Geometry check sheet. Reference: the model listing, model coordinates, mm. A direction names the side the tool comes from. Round coordinates to 2 decimals unless told otherwise and drop trailing zeros. Write each loop counter-clockwise with the first axis right and the second up, starting at its lowest first coordinate (ties: lowest second). Pieces come first, ordered by that corner, then holes. Notation, with made-up numbers: (68.25, -37.5) -> (91.25, -37.5) arc R18 ccw to (91.25, -17.5) -> close; hole circle Ø6 at (49.25, -13). An arc over 180 degrees is marked (long way). One line per question, with ' | ' between items.
```python
from build123d import *

# Parameters (mm, degrees)
SKETCH_1_R          = 17
EXTRUDE_1_DEPTH     = 5
SKETCH_2_R          = 2.8
CUT_EXTRUDE_1_DEPTH = 3
SKETCH_3_R          = 2.55
CUT_EXTRUDE_2_DEPTH = 6
SKETCH_7_R          = 1.55
CUT_EXTRUDE_4_DEPTH = 3


with BuildPart() as part:
    # 草图1 → 凸台-拉伸1 (new body)
    with BuildSketch(Plane.XY):
        Circle(SKETCH_1_R)
    extrude(amount=EXTRUDE_1_DEPTH)

    # 草图2 → 切除-拉伸1 (cut)
    with BuildSketch(Plane(origin=(0, 0, 0), x_dir=(-1, 0, 0), z_dir=(0, 0, -1))):
        with Locations((0, 8.75)):
            Circle(SKETCH_2_R)
        with Locations((7.577722283, -4.375)):
            Circle(SKETCH_2_R)
        with Locations((-7.577722283, -4.375)):
            Circle(SKETCH_2_R)
    extrude(amount=-CUT_EXTRUDE_1_DEPTH, mode=Mode.SUBTRACT)

    # 草图3 → 切除-拉伸2 (cut, through all)
    with BuildSketch(Plane(origin=(0, 0, 0), x_dir=(-1, 0, 0), z_dir=(0, 0, -1))):
        Circle(SKETCH_3_R)
    extrude(amount=-CUT_EXTRUDE_2_DEPTH, mode=Mode.SUBTRACT)

    # 草图7 → 切除-拉伸4 (cut, through all)
    with BuildSketch(Plane(origin=(0, 0, 3), x_dir=(-1, 0, 0), z_dir=(0, 0, -1))):
        with Locations((-7.577722283, -4.375)):
            Circle(SKETCH_7_R)
        with Locations((7.577722283, -4.375)):
            Circle(SKETCH_7_R)
        with Locations((0, 8.75)):
            Circle(SKETCH_7_R)
    extrude(amount=-CUT_EXTRUDE_4_DEPTH, mode=Mode.SUBTRACT)


solid = part.part
```
(1) Sectioned sample at B-B on x = 0. Record the cut outline in (y, z).
Resolved:
outline: (-17, 0) -> (-2.55, 0) -> (-2.55, 5) -> (-17, 5) -> close; (2.55, 0) -> (5.95, 0) -> (5.95, 3) -> (7.2, 3) -> (7.2, 5) -> (2.55, 5) -> close; (10.3, 3) -> (11.55, 3) -> (11.55, 0) -> (17, 0) -> (17, 5) -> (10.3, 5) -> close
(2) Sectioned sample at C-C on y = 9.5. Record the cut outline in (x, z), then the cut area to 3 significant figures.
Resolved:
outline: (-14.1, 0) -> (-2.7, 0) -> (-2.7, 3) -> (-1.36, 3) -> (-1.36, 5) -> (-14.1, 5) -> close; (1.36, 3) -> (2.7, 3) -> (2.7, 0) -> (14.1, 0) -> (14.1, 5) -> (1.36, 5) -> close | area: 119 mm2
(3) Sectioned sample at D-D on z = 4.2. Record the cut outline in (x, y) (3 decimals), then the cut area to 3 significant figures.
Resolved:
outline: circle Ø34 at (0, 0); hole circle Ø3.1 at (-7.578, -4.375); hole circle Ø5.1 at (0, 0); hole circle Ø3.1 at (0, 8.75); hole circle Ø3.1 at (7.578, -4.375) | area: 865 mm2
(4) Go/stop test with flat-tipped pins: pin 1 (4.5 mm diameter, centred on x = -7.5, y = -4.5, fed in from -Z); pin 2 (2 mm diameter, centred on y = 1.5, z = 2.5, fed in from -X). Record where each tip stops, or that it passes through.
Resolved:
pin 1: stops at z = 3 | pin 2: stops at x = -16.99
(5) Material ranges on line 1 (Y direction, x = -1, z = 1.25); line 2 (Y direction, x = -0.5, z = 3.2); line 3 (X direction, y = -5.5, z = 3.7), recorded low to high.
Resolved:
line 1: y = -16.97 to -2.35, 2.35 to 6.13, 11.37 to 16.97 | line 2: y = -16.99 to -2.5, 2.5 to 7.28, 10.22 to 16.99 | line 3: x = -16.09 to -8.64, -6.51 to 6.51, 8.64 to 16.09
(6) Sectioned sample at A-A on y = 0. Record the cut outline in (x, z), then the cut area to 4 significant figures.
Resolved:
outline: (-17, 0) -> (-2.55, 0) -> (-2.55, 5) -> (-17, 5) -> close; (2.55, 0) -> (17, 0) -> (17, 5) -> (2.55, 5) -> close | area: 144.5 mm2
(7) Access from +Z, -Z, +X, -X, +Y, -Y to the whole of each face (thin tool, end or side, straight path). Record for faces 1 (the cylindrical face through (-7.376, -2.838, 3.986)), 2 (the flat face through (-9, -6, 3)).
Resolved:
face 1: +Z, -Z | face 2: -Z
(8) Draft check along Y on faces 3 (the flat face through (4, 0, 5)), 4 (the cylindrical face through (9.139, 14.334, 2.465)), 5 (the flat face through (-1.2, 7.5, 3)), 6 (the flat face through (6, -6, 3)). Enter one of: +Y half, -Y half, draft (parallel to the pull), parting line (faces both ways), or undercut.
Resolved:
face 3: draft | face 4: parting line | face 5: undercut | face 6: undercut
